Can you work these out from the model? Positions are in its coordinate system, mm. A direction names the side the tool comes from. Coordinates: 2 decimals unless noted, no trailing zeros. Order: outer loops, then holes, each group sorted by start corner. A loop starts at its lowest first (then second) coordinate and runs counter-clockwise, first axis right, second up. Notation, with made-up numbers: (-29, 73.5) - (-8, 73.5) arc R28 cw to (-8, 107.5) - close; hole circle Ø9 at (-3.5, 49.5). An arc over 180 degrees is marked (long way). Use a Markdown table: item, result. Add a question column.
(1) If I drill on L1, parallel to Z at x = 1, y = 5.25; L2, parallel to Y at x = 0.75, z = -28; L3, parallel to X at y = 1.5, z = -17, over which ranges is the centre line in solid material (lowest first)? Write a range as [from, to].
(2) I want a section at D-D (z = -39). List the corners of the cut face in (x, y) for me.
(3) For pin 1 Ø4 at (x, z) = (-1, 2) entering from -Y; pin 2 Ø1 at (x, z) = (-5, -31) entering from -Y; pin 3 Ø0.8 at (y, z) = (5, -40.5) entering from -X, each with a flat end and sliding along its axis, tell me the tip position at first contact or that it passes through.
(4) I want a section at B-B (y = 0). List the corners of the cut face in (x, z) for me, and give its area (3 significant figures).
(5) I want a section at C-C (z = -26). List the corners of the cut face in (x, y) for me.
(6) On a 3-axis mill with a long thin cutter (end or side, diameter ignored), from which of +Z, -Z, +X, -X, +Y, -Y can I reach the whole of each face in a straight line? I mean faces 5 (the flat face through (-3.2, -5.6, 23)), 6 (the flat face through (-3, 5.7, 23)), 7 (the flat face through (-3.2, -5.6, -23)). Say none if no direction works.
(7) I want a section at A-A (z = -10). List the corners of the cut face in (x, y) for me.
(8) We'd pull the mould along X, two halves only. Please class faces 1 (the cylindrical face through (2.884, -5.545, -33.846)), 2 (the flat face through (0, 5, -32)), 3 (the flat face through (5.49, 2.99, -0.32)), 4 (the flat face through (-3.25, 5, -39)): pulls with the +X half, pulls with the -X half, needs draft (parallel to the pull), parting line crosses it, or undercut.
```python
from build123d import *

# Parameters (mm, degrees)
SKETCH1_R                = 6.25
BOSS_EXTRUDE1_DEPTH      = 37
BOSS_EXTRUDE1_DEPTH_BACK = 45
SKETCH4_W                = 6.5
SKETCH4_H                = 5
CUT_EXTRUDE1_DEPTH       = 13
BOSS_EXTRUDE2_DEPTH      = 46
FILLET1_R                = 3


with BuildPart() as part:
    # Sketch1 → Boss-Extrude1 (new body, two sides)
    with BuildSketch(Plane.XY) as boss_extrude1_sk:
        Circle(SKETCH1_R)
    extrude(amount=BOSS_EXTRUDE1_DEPTH)
    extrude(boss_extrude1_sk.sketch, amount=-BOSS_EXTRUDE1_DEPTH_BACK)

    # Sketch4 → Cut-Extrude1 (cut)
    with BuildSketch(Plane(origin=(0, 0, -45), x_dir=(-1, 0, 0), z_dir=(0, 0, -1))):
        with Locations((0, 6.25)):
            Rectangle(SKETCH4_W, SKETCH4_H)
    extrude(amount=-CUT_EXTRUDE1_DEPTH, mode=Mode.SUBTRACT)

    # Sketch5 → Boss-Extrude2 (add)
    with BuildSketch(Plane.XY.offset(-23)):
        Polygon((3.732897661, 6.176472163), (-3.482532969, 6.321020286), (-7.21543063, 0.144548123), (-3.732897661, -6.176472163), (3.482532969, -6.321020286), (7.21543063, -0.144548123), align=None)
    extrude(amount=BOSS_EXTRUDE2_DEPTH)

    # Fillet1
    fillet1_edges = [part.edges().sort_by_distance(p)[0] for p in [
        (7.21543063, -0.144548123, 0),
        (3.732897661, 6.176472163, 0),
        (-3.482532969, 6.321020286, 0),
        (-7.21543063, 0.144548123, 0),
        (-3.732897661, -6.176472163, 0),
        (3.482532969, -6.321020286, 0),
    ]]
    fillet(fillet1_edges, radius=FILLET1_R)


solid = part.part
```
Answers follow:
| question | item | result |
|---|---|---|
| 1 | L1 | z = [-32, 37] |
| 1 | L2 | y = [-6.2, 6.2] |
| 1 | L3 | x = [-6.39, 6.31] |
| 2 | outline | (-3.25, 3.75) - (-3.25, 5.34) arc R6.25 ccw (long way) to (3.25, 5.34) - (3.25, 3.75) - close |
| 3 | pin 1 | stops at y = -6.27 |
| 3 | pin 2 | stops at y = -4.34 |
| 3 | pin 3 | stops at x = -4.23 |
| 4 | outline | (-6.75, -23) - (-6.25, -23) - (-6.25, -45) - (6.25, -45) - (6.25, -23) - (6.75, -23) - (6.75, 23) - (6.25, 23) - (6.25, 37) - (-6.25, 37) - (-6.25, 23) - (-6.75, 23) - close |
| 4 | area | 1,070 mm² |
| 5 | outline | circle Ø12.5 at (0, 0) |
| 6 | face 5 | +Z, -X, -Y |
| 6 | face 6 | +Z, -X, +Y |
| 6 | face 7 | -Z, -X, -Y |
| 7 | outline | (-6.38, -1.37) - (-4.57, -4.66) arc R3 ccw to (-2, -6.21) - (1.75, -6.29) arc R3 ccw to (4.38, -4.84) - (6.32, -1.63) arc R3 ccw to (6.38, 1.37) - (4.57, 4.66) arc R3 ccw to (2, 6.21) - (-1.75, 6.29) arc R3 ccw to (-4.38, 4.84) - (-6.32, 1.63) arc R3 ccw to start |
| 8 | face 1 | parting line crosses it |
| 8 | face 2 | undercut |
| 8 | face 3 | pulls with the +X half |
| 8 | face 4 | undercut |
